CAD build for the part. Positions are in the model's coordinates, mm. Coordinates: 2 decimals unless noted, no trailing zeros. Order: outer loops, then holes, each group sorted by start corner. A loop starts at its lowest first (then second) coordinate and runs counter-clockwise, first axis right, second up. Notation, with made-up numbers: M -25,31 L 0,31 A21 ccw 0,55 Z; hole C -22,76 d10. An arc over 180 degrees is marked long. Write item = value, one per line. Start each with the question number.
Autodesk Inventor part; units mm, degrees
ref_plane "YZ Plane" through (0, 0, 0) normal (1, 0, 0) x (0, 1, 0)
ref_plane "XZ Plane" through (0, 0, 0) normal (0, 1, 0) x (-1, 0, 0)
ref_plane "XY Plane" through (0, 0, 0) normal (0, 0, 1) x (1, 0, 0)
sketch "Sketch1" plane through (0, 0, 0) normal (0, 0, 1) x (1, 0, 0)
  line L0 (6.35, 3.6662) -> (6.35, -3.6662)
  line L1 (6.35, -3.6662) -> (0, -7.3323)
  line L2 (0, -7.3323) -> (-6.35, -3.6662)
  line L3 (-6.35, -3.6662) -> (-6.35, 3.6662)
  line L4 (-6.35, 3.6662) -> (0, 7.3323)
  line L5 (0, 7.3323) -> (6.35, 3.6662)
  circle A0 centre (0, 0) radius 1.4224
  dimension "d0" = 12.7
  dimension "d3" = 2.8448
extrude "Extrusion1" add sketch "Sketch1" against normal blind 355.6
properties part number "SHAFT,HEX,0.500in,DRIVE,ELEVATOR" material "Steel, Alloy"
1. Slice it at A-A (z = -180.5). Write the cut outline in (x, y).
2. Mould opens along Z. For faces 1 (the flat face through (3.131, 5.525, -175.311)), 2 (the flat face through (0, -2, 0)), 3 (the flat face through (0, -2, -355.6)) say: released by +Z, released by -Z, zero draft, split by the parting line, or undercut.
3. Slice it at B-B (x = -4.25). Write the cut outline in (y, z).
4. Probe L1, parallel to Y at x = 0, z = -79; L2, parallel to X at y = -0.25, z = -193; L3, parallel to X at y = -6.5, z = -238. List the from-to ranges inside material, lowest first.
5. Flat gauge pin, fed straight in: pin 1 (1.5 mm diameter, centred on x = -3.5, z = -210.5, fed in from +Y). Where does the tip first touch, or does it go through?
Calculated:
q1.outline = M -6.35,-3.67 L 0,-7.33 L 6.35,-3.67 L 6.35,3.67 L 0,7.33 L -6.35,3.67 Z; hole C 0,0 d2.84
q2.face_1 = zero draft
q2.face_2 = released by +Z
q2.face_3 = released by -Z
q3.outline = M -4.88,-355.6 L 4.88,-355.6 L 4.88,0 L -4.88,0 Z
q4.L1 = -7.33 to -1.42, 1.42 to 7.33
q4.L2 = -6.35 to -1.4, 1.4 to 6.35
q4.L3 = -1.44 to 1.44
q5.pin_1 = 5.74
